CAD build for the part. Positions are in the model's coordinates, mm. Give positions to 0.01 mm unless a question says otherwise; leave off trailing zeros. Loops run counter-clockwise (first coordinate to the right, second up) from the corner with the lowest first, then second, coordinate; pieces in that order, holes last.
```python
from build123d import *

# Parameters (mm, degrees)
SKETCH1_W           = 6
SKETCH1_H           = 9
BOSS_EXTRUDE1_DEPTH = 1
SKETCH2_W           = 1
SKETCH2_H           = 3
BOSS_EXTRUDE2_DEPTH = 100
SKETCH3_W           = 1
SKETCH3_H           = 9
BOSS_EXTRUDE3_DEPTH = 50
SKETCH4_W           = 51
SKETCH4_H           = 9
BOSS_EXTRUDE4_DEPTH = 0.5
BOSS_EXTRUDE5_DEPTH = 0.5


with BuildPart() as part:
    # Sketch1 → Boss-Extrude1 (new body)
    with BuildSketch(Plane.XY):
        with Locations((3, 4.5)):
            Rectangle(SKETCH1_W, SKETCH1_H)
    extrude(amount=BOSS_EXTRUDE1_DEPTH)

    # Sketch2 → Boss-Extrude2 (add)
    with BuildSketch(Plane(origin=(0, 0, 0), x_dir=(-1, 0, 0), z_dir=(0, 0, -1))):
        with Locations((-0.5, 1.5)):
            Rectangle(SKETCH2_W, SKETCH2_H)
        with Locations((-0.5, 7.5)):
            Rectangle(SKETCH2_W, SKETCH2_H)
    extrude(amount=BOSS_EXTRUDE2_DEPTH)

    # Sketch3 → Boss-Extrude3 (add)
    with BuildSketch(Plane(origin=(0, 0, 0), x_dir=(-1, 0, 0), z_dir=(0, 0, -1))):
        with Locations((-5.5, 4.5)):
            Rectangle(SKETCH3_W, SKETCH3_H)
    extrude(amount=BOSS_EXTRUDE3_DEPTH)

    # Sketch4 → Boss-Extrude4 (add)
    with BuildSketch(Plane(origin=(6, 0, 0), x_dir=(0, 0, -1), z_dir=(1, 0, 0))):
        with Locations((24.5, 4.5)):
            Rectangle(SKETCH4_W, SKETCH4_H)
    extrude(amount=BOSS_EXTRUDE4_DEPTH)

    # Sketch5 → Boss-Extrude5 (add)
    with BuildSketch(Plane.ZY):
        Polygon((1, 9), (-100, 9), (-100, 6), (0, 6), (0, 3), (-100, 3), (-100, 0), (1, 0), align=None)
    extrude(amount=BOSS_EXTRUDE5_DEPTH)


solid = part.part
```
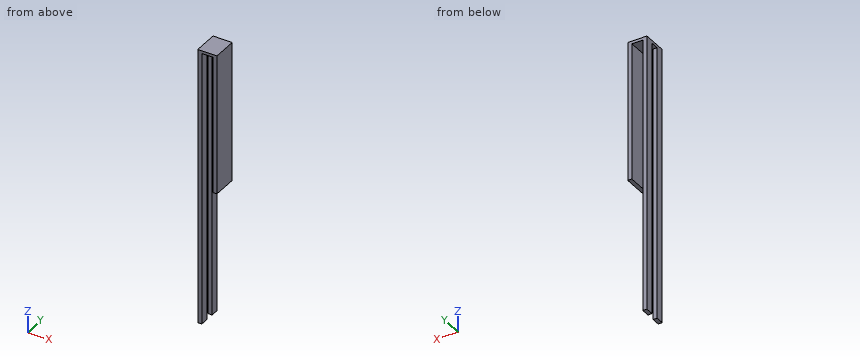
1. Saw through at C-C, the plane y = 7.75. List the corners of the cut face in (x, z), and give its area (3 significant figures).
Responses:
outline: (-0.5, -100) - (1, -100) - (1, 0) - (5, 0) - (5, -50) - (6.5, -50) - (6.5, 1) - (-0.5, 1) - close
area: 232 mm2
2. Saw through at B-B, the plane z = -15. List the corners of the cut face in (x, y).
Responses:
outline: (-0.5, 0) - (1, 0) - (1, 3) - (-0.5, 3) - close; (-0.5, 6) - (1, 6) - (1, 9) - (-0.5, 9) - close; (5, 0) - (6.5, 0) - (6.5, 9) - (5, 9) - close
3. Saw through at D-D, the plane x = 2.25. List the corners of the cut face in (y, z).
Responses:
outline: (0, 0) - (9, 0) - (9, 1) - (0, 1) - close
4. Drop flat-ended pins along their axis: pin 1 (2 mm diameter, centred on x = 5, y = 2, fed in from -Z); pin 2 (3.5 mm diameter, centred on y = 1.5, z = -55.5, fed in from +X); pin 3 (1 mm diameter, centred on y = 5, z = -61, fed in from -X). Give the stop position or say it passes through.
Responses:
pin 1: stops at z = -50
pin 2: stops at x = 1
pin 3: passes through
5. Saw through at A-A, the plane z = -62. List the corners of the cut face in (x, y).
Responses:
outline: (-0.5, 0) - (1, 0) - (1, 3) - (-0.5, 3) - close; (-0.5, 6) - (1, 6) - (1, 9) - (-0.5, 9) - close
6. Probe line 1 along Y through (x, z) = (0, -14); line 2 along X through (y, z) = (7.5, -94.5); line 3 along Z through (x, y) = (2.5, 6.5). List the from-to ranges inside material, lowest first.
Responses:
line 1: y = 0 to 3, 6 to 9
line 2: x = -0.5 to 1
line 3: z = 0 to 1
